from build123d import *

# Parameters (mm, degrees)
SKETCH_1_W          = 46.5
SKETCH_1_H          = 91
SKETCH_1_R          = 1.6
EXTRUDE_1_DEPTH     = 50
HOLE_WIZARD_1_D     = 4
HOLE_WIZARD_2_D     = 4
HOLE_WIZARD_2_DEPTH = 100


with BuildPart() as part:
    # 草图1 → 凸台-拉伸1 (new body)
    with BuildSketch(Plane(origin=(0, 0, 0), x_dir=(1, 0, 0), z_dir=(0, 1, 0))):
        Rectangle(SKETCH_1_W, SKETCH_1_H)
        with Locations(Location((20, 43.5, 0), (0, 0, 270))):
            Circle(SKETCH_1_R, mode=Mode.SUBTRACT)
        with Locations(Location((-20, 43.5, 0), (0, 0, 90))):
            Circle(SKETCH_1_R, mode=Mode.SUBTRACT)
        with Locations(Location((-20, -40.5, 0), (0, 0, 270))):
            Circle(SKETCH_1_R, mode=Mode.SUBTRACT)
    extrude(amount=EXTRUDE_1_DEPTH)

    # 孔1 (through all)
    with Locations(Plane(origin=(0, 50, 0), x_dir=(1, 0, 0), z_dir=(0, 1, 0))):
        with Locations((19.042, -19.406)):
            Hole(HOLE_WIZARD_1_D / 2)

    # 孔2
    with Locations(Plane(origin=(0, 50, 0), x_dir=(1, 0, 0), z_dir=(0, 1, 0))):
        with Locations((19.042, 33.984), (-20.583, 33.984), (-20.583, -19.406)):
            Hole(HOLE_WIZARD_2_D / 2, depth=HOLE_WIZARD_2_DEPTH)


solid = part.part
Could you check a few things on this model? Use its own coordinates, in mm. Round coordinates to 2 decimals unless told otherwise and drop trailing zeros. Order: outer loops, then holes, each group sorted by start corner. A loop starts at its lowest first (then second) coordinate and runs counter-clockwise, first axis right, second up.
Q1. Thinking about a two-plate mould opening in Z: for faces 1 (the face through (21.586, 24.65, -43.708)), 2 (the face through (0, 25, 45.5)), 3 (the face through (0, 50, -1)), 4 (the face through (0, 25, -45.5)), which applies, released by +Z, released by -Z, zero draft, split by the parting line, or undercut?
Geometry says:
face 1: undercut
face 2: released by +Z
face 3: zero draft
face 4: released by -Z
Q2. Imagine slicing it at C-C, the plane y = 30.5. List the corners of the cut face in (x, z) for me, then the cut area to 3 significant figures.
Geometry says:
outline: (-23.25, -45.5) - (23.25, -45.5) - (23.25, 45.5) - (-23.25, 45.5) - close; hole circle Ø4 at (-20.58, -33.98); hole circle Ø4 at (-20.58, 19.41); hole circle Ø3.2 at (-20, -43.5); hole circle Ø3.2 at (-20, 40.5); hole circle Ø4 at (19.04, -33.98); hole circle Ø4 at (19.04, 19.41); hole circle Ø3.2 at (20, -43.5)
area: 4,160 mm2
Q3. Imagine slicing it at A-A, the plane z = 40.5. List the corners of the cut face in (x, y) for me, then the cut area to 4 significant figures.
Geometry says:
outline: (-23.25, 0) - (-21.6, 0) - (-21.6, 50) - (-23.25, 50) - close; (-18.4, 0) - (23.25, 0) - (23.25, 50) - (-18.4, 50) - close
area: 2,165 mm2
Q4. Imagine slicing it at D-D, the plane z = -43.5. List the corners of the cut face in (x, y) for me, then the cut area to 4 significant figures.
Geometry says:
outline: (-23.25, 0) - (-21.6, 0) - (-21.6, 50) - (-23.25, 50) - close; (-18.4, 0) - (18.4, 0) - (18.4, 50) - (-18.4, 50) - close; (21.6, 0) - (23.25, 0) - (23.25, 50) - (21.6, 50) - close
area: 2,005 mm2
Q5. Please list where these lines run through material, in increasing order: probe 1 along X at (y, z) = (30, -43); probe 2 along Z at (x, y) = (17.5, 29.5); probe 3 along Z at (x, y) = (-19, 8).
Geometry says:
probe 1: x = -23.25 to -21.52, -18.48 to 18.48, 21.52 to 23.25
probe 2: z = -45.5 to -35.26, -32.71 to 18.13, 20.68 to 45.5
probe 3: z = -45.5 to -44.75, -42.25 to -35.21, -32.76 to 18.18, 20.63 to 39.25, 41.75 to 45.5
Q6. Imagine slicing it at B-B, the plane x = -20. List the corners of the cut face in (y, z) for me, then the cut area to 3 significant figures.
Geometry says:
outline: (0, -45.5) - (50, -45.5) - (50, -45.1) - (0, -45.1) - close; (0, -41.9) - (50, -41.9) - (50, -35.9) - (0, -35.9) - close; (0, -32.07) - (50, -32.07) - (50, 17.49) - (0, 17.49) - close; (0, 21.32) - (50, 21.32) - (50, 38.9) - (0, 38.9) - close; (0, 42.1) - (50, 42.1) - (50, 45.5) - (0, 45.5) - close
area: 3,850 mm2
